from build123d import *

# Parameters (mm, degrees)
F0_W     = 97.442076
F0_H     = 40
F1_DEPTH = 15
F2_R     = 12.912954
F3_DEPTH = 100
F4_R     = 7.192075
F5_DEPTH = 1000


with BuildPart() as f1:
    # F0 (on Front) → F1 (new body, symmetric)
    with BuildSketch(Plane.XZ):
        Rectangle(F0_W, F0_H)
    extrude(amount=F1_DEPTH, both=True)

    # F2 (on face) → F3 (cut)
    with BuildSketch(Plane.XZ.offset(15)):
        with Locations((-33.078179, 0)):
            Circle(F2_R)
    extrude(amount=-F3_DEPTH, mode=Mode.SUBTRACT)

    # F4 (on face) → F5 (cut)
    with BuildSketch(Plane(origin=(-48.721038, 0, 0), x_dir=(0, -1, 0), z_dir=(-1, 0, 0))):
        Circle(F4_R)
    extrude(amount=-F5_DEPTH, mode=Mode.SUBTRACT)


solid = f1.part
Part model, mm, in its own coordinate system. Coordinates: 2 decimals unless noted, no trailing zeros. Order: outer loops, then holes, each group sorted by start corner. A loop starts at its lowest first (then second) coordinate and runs counter-clockwise, first axis right, second up. Notation, with made-up numbers: M 75.25,-16.5 L 129.25,-16.5 A19 cw 129.25,7.5 Z; hole C 66.5,78 d7. An arc over 180 degrees is marked long. Use a Markdown table: item, result.
(1) Flat gauge pins, fed straight in: pin 1 (12 mm diameter, centred on x = -26, z = -9.5, fed in from -Y); pin 2 (1.5 mm diameter, centred on y = 0.5, z = 5.5, fed in from +X). Where does each tip first touch, or does it go through?
A:
| item | result |
|---|---|
| pin 1 | stops at y = -15 |
| pin 2 | passes through |
(2) Pull direction X, two halves, no side cores. Call faces 1 (the flat face through (-1, 15, 0)), 2 (the cylindrical face through (-43.325, -0.21, -7.857)), 3 (the flat face through (48.721, -7, -5)): released by +X, released by -X, zero draft, split by the parting line, or undercut.
A:
| item | result |
|---|---|
| face 1 | zero draft |
| face 2 | undercut |
| face 3 | released by +X |
(3) Cut at C-C on x = -25. Write the cut outline in (y, z), then the cut area to 3 significant figures.
A:
| item | result |
|---|---|
| outline | M -15,-20 L 15,-20 L 15,-10.07 L -15,-10.07 Z; M -15,10.07 L 15,10.07 L 15,20 L -15,20 Z |
| area | 596 mm^2 |
(4) Probe L1, parallel to Y at x = -47, z = 0; L2, parallel to Z at x = 0.5, y = -0.5; L3, parallel to X at y = 12, z = 7. List the from-to ranges inside material, lowest first.
A:
| item | result |
|---|---|
| L1 | y = -15 to -7.19, 7.19 to 15 |
| L2 | z = -20 to -7.17, 7.17 to 20 |
| L3 | x = -48.72 to -43.93, -22.23 to 48.72 |
(5) Cut at A-A on y = 0. Write the cut outline in (x, z).
A:
| item | result |
|---|---|
| outline | M -48.72,-20 L 48.72,-20 L 48.72,-7.19 L -22.35,-7.19 A12.91 cw -43.8,-7.19 L -48.72,-7.19 Z; M -48.72,7.19 L -43.8,7.19 A12.91 cw -22.35,7.19 L 48.72,7.19 L 48.72,20 L -48.72,20 Z |
(6) Cut at D-D on z = -5. Write the cut outline in (x, y).
A:
| item | result |
|---|---|
| outline | M -48.72,-15 L -44.98,-15 L -44.98,-5.17 L -48.72,-5.17 Z; M -48.72,5.17 L -44.98,5.17 L -44.98,15 L -48.72,15 Z; M -21.17,-15 L 48.72,-15 L 48.72,-5.17 L -21.17,-5.17 Z; M -21.17,5.17 L 48.72,5.17 L 48.72,15 L -21.17,15 Z |
(7) Cut at B-B on z = -12. Write the cut outline in (x, y), then the cut area to 3 significant figures.
A:
| item | result |
|---|---|
| outline | M -48.72,-15 L -37.85,-15 L -37.85,15 L -48.72,15 Z; M -28.31,-15 L 48.72,-15 L 48.72,15 L -28.31,15 Z |
| area | 2,640 mm^2 |
